The model under review builds one solid part; all positions refer to its coordinate system, in mm. Give positions to 0.01 mm unless a question says otherwise; leave off trailing zeros. Loops run counter-clockwise (first coordinate to the right, second up) from the corner with the lowest first, then second, coordinate; pieces in that order, holes last. Notation, with made-up numbers: (-12.5, 30.25) - (5.5, 30.25) arc R16 cw to (5.5, 44.25) - close; hole circle Ø8 at (80, 64). An arc over 180 degrees is marked (long way). Answer as a JSON object with one key per item and string values.
from build123d import *

# Parameters (mm, degrees)
SKETCH1_W           = 100
SKETCH1_H           = 102.3
BOSS_EXTRUDE1_DEPTH = 5
SKETCH4_R           = 2.2
CUT_EXTRUDE1_DEPTH  = 5
LPATTERN1_COUNT     = 2
LPATTERN1_PITCH     = 60
SKETCH6_R           = 1.6
SKETCH6_R_2         = 11.5
CUT_EXTRUDE4_DEPTH  = 10
SKETCH8_R           = 2.2
CUT_EXTRUDE5_DEPTH  = 10
SKETCH9_R           = 2.5
CUT_EXTRUDE6_DEPTH  = 10


with BuildPart() as part:
    # Sketch1 → Boss-Extrude1 (new body)
    with BuildSketch(Plane.XY):
        Rectangle(SKETCH1_W, SKETCH1_H)
    extrude(amount=BOSS_EXTRUDE1_DEPTH)

    # Sketch4 → Cut-Extrude1 (cut)
    with BuildSketch(Plane.XY.offset(5)):
        with Locations((39, -22.15)):
            Circle(SKETCH4_R)
        with Locations((39, -46.15)):
            Circle(SKETCH4_R)
        with Locations((21, -46.15)):
            Circle(SKETCH4_R)
        with Locations((21, -22.15)):
            Circle(SKETCH4_R)
    cut_extrude1 = extrude(amount=-CUT_EXTRUDE1_DEPTH, mode=Mode.SUBTRACT)

    # LPattern1: Cut-Extrude1 ×2
    with Locations(*[(-i * LPATTERN1_PITCH, 0, 0) for i in range(1, LPATTERN1_COUNT)]):
        add(cut_extrude1, mode=Mode.SUBTRACT)

    # Sketch6 → Cut-Extrude4 (cut)
    with BuildSketch(Plane.XY.offset(5)):
        with Locations((-44.499679494, 32.649679494)):
            Circle(SKETCH6_R)
        with Locations((-13.49967952, 32.650961002)):
            Circle(SKETCH6_R)
        with Locations((-44.499680011, 1.649679494)):
            Circle(SKETCH6_R)
        with Locations((-13.5, 1.65)):
            Circle(SKETCH6_R)
        with Locations((-29, 17.15)):
            Circle(SKETCH6_R_2)
    extrude(amount=-CUT_EXTRUDE4_DEPTH, mode=Mode.SUBTRACT)

    # Sketch8 → Cut-Extrude5 (cut)
    with BuildSketch(Plane.XY.offset(5)):
        with Locations((-4, 46.15)):
            Circle(SKETCH8_R)
        with Locations((14, 46.15)):
            Circle(SKETCH8_R)
        with Locations((-4, 22.15)):
            Circle(SKETCH8_R)
        with Locations((14, 22.15)):
            Circle(SKETCH8_R)
    extrude(amount=-CUT_EXTRUDE5_DEPTH, mode=Mode.SUBTRACT)

    # Sketch9 → Cut-Extrude6 (cut)
    with BuildSketch(Plane.XY.offset(5)):
        with Locations((-39, -6.85)):
            Circle(SKETCH9_R)
        with Locations((-19, -6.85)):
            Circle(SKETCH9_R)
    extrude(amount=-CUT_EXTRUDE6_DEPTH, mode=Mode.SUBTRACT)


solid = part.part
Q1. Consider section D-D, the plane y = 46.15. State the section outline as (x, z) points, plus the area to 3 significant figures.
Results:
{"outline": "(-50, 0) - (-6.2, 0) - (-6.2, 5) - (-50, 5) - close; (-1.8, 0) - (11.8, 0) - (11.8, 5) - (-1.8, 5) - close; (16.2, 0) - (50, 0) - (50, 5) - (16.2, 5) - close", "area": "456 mm^2"}
Q2. Consider section C-C, the plane y = -22.15. State the section outline as (x, z) points.
Results:
{"outline": "(-50, 0) - (-41.2, 0) - (-41.2, 5) - (-50, 5) - close; (-36.8, 0) - (-23.2, 0) - (-23.2, 5) - (-36.8, 5) - close; (-18.8, 0) - (18.8, 0) - (18.8, 5) - (-18.8, 5) - close; (23.2, 0) - (36.8, 0) - (36.8, 5) - (23.2, 5) - close; (41.2, 0) - (50, 0) - (50, 5) - (41.2, 5) - close"}
Q3. The part is to be moulded in two halves that separate along Y. For faces 1 (the face through (50, -1, 2)), 2 (the face through (-1, 51.15, 2)), 3 (the face through (-18.9, -21.5, 2.5)), say which applies: +Y half, -Y half, draft (parallel to the pull), parting line (faces both ways), or undercut.
Results:
{"face 1": "draft", "face 2": "+Y half", "face 3": "undercut"}
Q4. To check wall thickness, follow probe 1 along Y at (x, z) = (39, 2.1); probe 2 along Y at (x, z) = (-39, 2.5); probe 3 along X at (y, z) = (2, 4). State the ranges of each line that lie inside material, in increasing order. Write a range as [from, to].
Results:
{"probe 1": "y = [-51.15, -48.35], [-43.95, -24.35], [-19.95, 51.15]", "probe 2": "y = [-51.15, -48.35], [-43.95, -24.35], [-19.95, -9.35], [-4.35, 11.47], [22.83, 51.15]", "probe 3": "x = [-50, -46.06], [-42.94, -15.06], [-11.94, 50]"}
Q5. Consider section B-B, the plane x = -29. State the section outline as (y, z) points, plus the area to 4 significant figures.
Results:
{"outline": "(-51.15, 0) - (5.65, 0) - (5.65, 5) - (-51.15, 5) - close; (28.65, 0) - (51.15, 0) - (51.15, 5) - (28.65, 5) - close", "area": "396.5 mm^2"}
Q6. Consider section A-A, the plane x = -4. State the section outline as (y, z) points.
Results:
{"outline": "(-51.15, 0) - (19.95, 0) - (19.95, 5) - (-51.15, 5) - close; (24.35, 0) - (43.95, 0) - (43.95, 5) - (24.35, 5) - close; (48.35, 0) - (51.15, 0) - (51.15, 5) - (48.35, 5) - close"}
